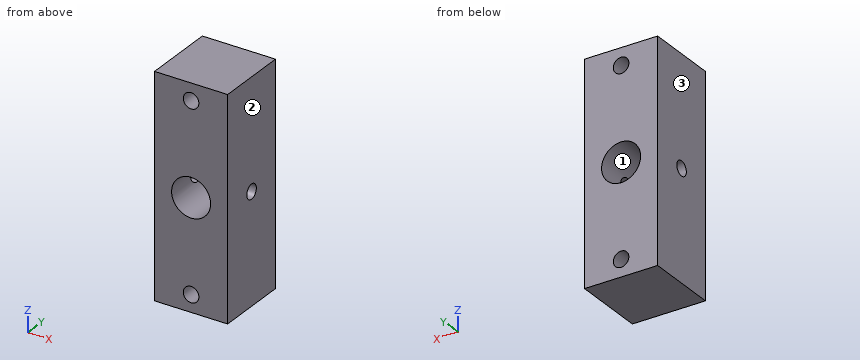
```python
from build123d import *

# Parameters (mm, degrees)
SKETCH_1_W          = 15
SKETCH_1_H          = 45
SKETCH_1_R          = 4
SKETCH_1_R_2        = 1.6
EXTRUDE_1_DEPTH     = 7.5
SKETCH_2_R          = 1.5
CUT_EXTRUDE_1_DEPTH = 29.062430401


with BuildPart() as part:
    # 草图1 → 凸台-拉伸1 (new, symmetric)
    with BuildSketch(Plane(origin=(0, 0, 0), x_dir=(1, 0, 0), z_dir=(0, 1, 0))):
        Rectangle(SKETCH_1_W, SKETCH_1_H)
        with Locations(Location((0, 0, 0), (0, 0, 270))):
            Circle(SKETCH_1_R, mode=Mode.SUBTRACT)
        with Locations(Location((0, 19, 0), (0, 0, 270))):
            Circle(SKETCH_1_R_2, mode=Mode.SUBTRACT)
        with Locations(Location((0, -19, 0), (0, 0, 90))):
            Circle(SKETCH_1_R_2, mode=Mode.SUBTRACT)
    extrude(amount=EXTRUDE_1_DEPTH, both=True)

    # 草图2 → 切除-拉伸1 (cut, through all)
    with BuildSketch(Plane(origin=(7.5, 0, 0), x_dir=(0, 0, -1), z_dir=(1, 0, 0))):
        Circle(SKETCH_2_R)
    extrude(amount=-CUT_EXTRUDE_1_DEPTH, mode=Mode.SUBTRACT)


solid = part.part
```
Source: CAD feature listing. Evaluate the final solid. Frame: model axes, mm. Face numbers are marked on the shaded views. Give positions to 0.01 mm unless a question says otherwise; leave off trailing zeros. Loops run counter-clockwise (first coordinate to the right, second up) from the corner with the lowest first, then second, coordinate; pieces in that order, holes last. Notation, with made-up numbers: (8, 15) - (46, 15) arc R14 cw to (46, 23) - close; hole circle Ø11 at (79, 72.25). An arc over 180 degrees is marked (long way). Use CSV: the item, a comma, the result in double quotes. Start each with the question number.
1. Section D-D (z = 0). Output: boundary loops of the cut face in (x, y), then the cut area to 3 significant figures.
2. Section A-A (y = 0). Output: boundary loops of the cut face in (x, z), then the cut area to 3 significant figures.
3. Section B-B (z = 19). Output: boundary loops of the cut face in (x, y), then the cut area to 3 significant figures.
4. Pin query (flat end, axial travel): pin 1 (6.5 mm diameter, centred on x = 0, z = 0, fed in from +Y). Return the tip coordinate at first contact, or that it passes through.
5. Section C-C (x = 3.25). Output: boundary loops of the cut face in (y, z).
6. Ray query, L1, parallel to Y at x = 6.5, z = 0; L2, parallel to X at y = -2, z = 0; L3, parallel to Z at x = -5.6, y = 0. Return the intervals inside material, ascending.
7. Draft query along X for the marked faces 1, 2 and 3. Return one class per face: +X half, -X half, draft (parallel to the pull), parting line (faces both ways), or undercut.
Response:
1,outline,"(-7.5, -7.5) - (-4, -7.5) - (-4, -1.5) - (-7.5, -1.5) - close; (-7.5, 1.5) - (-4, 1.5) - (-4, 7.5) - (-7.5, 7.5) - close; (4, -7.5) - (7.5, -7.5) - (7.5, -1.5) - (4, -1.5) - close; (4, 1.5) - (7.5, 1.5) - (7.5, 7.5) - (4, 7.5) - close"
1,area,"84.0 mm²"
2,outline,"(-7.5, -22.5) - (7.5, -22.5) - (7.5, -1.5) - (3.71, -1.5) arc R4 cw to (-3.71, -1.5) - (-7.5, -1.5) - close; (-7.5, 1.5) - (-3.71, 1.5) arc R4 cw to (3.71, 1.5) - (7.5, 1.5) - (7.5, 22.5) - (-7.5, 22.5) - close; hole circle Ø3.2 at (0, -19); hole circle Ø3.2 at (0, 19)"
2,area,"587 mm²"
3,outline,"(-7.5, -7.5) - (-1.6, -7.5) - (-1.6, 7.5) - (-7.5, 7.5) - close; (1.6, -7.5) - (7.5, -7.5) - (7.5, 7.5) - (1.6, 7.5) - close"
3,area,"177 mm²"
4,pin 1,"through"
5,outline,"(-7.5, -22.5) - (7.5, -22.5) - (7.5, -2.33) - (-7.5, -2.33) - close; (-7.5, 2.33) - (7.5, 2.33) - (7.5, 22.5) - (-7.5, 22.5) - close"
6,L1,"-7.5 to -1.5, 1.5 to 7.5"
6,L2,"-7.5 to -4, 4 to 7.5"
6,L3,"-22.5 to -1.5, 1.5 to 22.5"
7,face 1,"undercut"
7,face 2,"+X half"
7,face 3,"-X half"
